Autodesk Inventor part; units mm, degrees
ref_plane "YZ Plane" through (0, 0, 0) normal (1, 0, 0) x (0, 1, 0)
ref_plane "XZ Plane" through (0, 0, 0) normal (0, 1, 0) x (-1, 0, 0)
ref_plane "XY Plane" through (0, 0, 0) normal (0, 0, 1) x (1, 0, 0)
sketch "Sketch1" plane through (0, 0, 0) normal (0, 1, 0) x (-1, 0, 0)
  line L0 (0, 0) -> (325, 0)
  line L1 (325, 0) -> (325, -10)
  line L2 (325, -10) -> (0, -10)
  line L3 (0, -10) -> (0, 0)
  dimension "d0" = 325
  dimension "d1" = 10
extrude "Extrusion1" add sketch "Sketch1" along normal blind 40
sketch "Sketch4" plane through (-325, 0, 0) normal (0, 0, 1) x (1, 0, 0)
  line L0 (325, 0) -> (0, 0)
  line L1 (325, 0) -> (325, 40)
  line L2 (0, 0) -> (325, 0)
  line L3 (325, 0) -> (325, 8)
  line L4 (325, 8) -> (0, 8)
  line L5 (0, 8) -> (0, 0)
  dimension "d34" = 8
extrude "Extrusion3" add sketch "Sketch4" along normal blind 20
sketch "Sketch5" plane through (-325, 40, 0) normal (0, 0, 1) x (1, 0, 0)
  circle A0 centre (320, -25) radius 1.5
  circle A1 centre (320, -15) radius 1.5
  line L0 (325, -32) -> (325, 0)
  line L1 (0, 0) -> (325, 0)
  circle A2 centre (5, -15) radius 1.5
  circle A3 centre (5, -25) radius 1.5
  line L2 (0, -32) -> (0, 0)
  point P0 (325, -40)
  point P1 (325, -27)
  point P2 (0, -27)
  dimension "d39" = 3
  dimension "d40" = 3
  dimension "d41" = 5
  dimension "d42" = 5
  dimension "d43" = 10
  dimension "d44" = 15
  dimension "d45" = 3
  dimension "d46" = 3
  dimension "d47" = 10
  dimension "d48" = 15
  dimension "d49" = 5
  dimension "d50" = 5
extrude "Extrusion4" cut sketch "Sketch5" against normal blind 20
thread "Thread1"
thread "Thread2"
thread "Thread3"
thread "Thread4"
sketch "Sketch8" plane through (0, 0, -10) normal (0, 0, -1) x (-1, 0, 0)
  line L0 (0, 40) -> (325, 40)
  line L1 (12.5, 37) -> (312.5, 37)
  line L2 (312.5, 37) -> (312.5, 0)
  line L3 (312.5, 0) -> (12.5, 0)
  line L4 (12.5, 0) -> (12.5, 37)
  line L5 (0, 0) -> (0, 40)
  line L6 (325, 0) -> (325, 40)
  point P0 (312.5, 18.5)
  dimension "d67" = 300
  dimension "d68" = 37
  dimension "d69" = 12.5
  dimension "d70" = 12.5
  dimension "d71" = 3
extrude "Extrusion5" add sketch "Sketch8" along normal blind 5
sketch "Sketch9" plane through (-325, 40, 0) normal (0, 0, 1) x (1, 0, 0)
  circle A0 centre (57.4993, -19.9899) radius 10
  circle A1 centre (87.4993, -19.9899) radius 10
  circle A2 centre (117.4993, -19.9899) radius 10
  circle A3 centre (147.4993, -19.9899) radius 10
  circle A4 centre (177.4993, -19.9899) radius 10
  circle A5 centre (207.4993, -19.9899) radius 10
  circle A6 centre (237.4993, -19.9899) radius 10
  circle A7 centre (267.4993, -19.9899) radius 10
  line L0 (-0.0007, -39.9899) -> (-0.0007, 0.0101)
  line L1 (324.9993, -39.9899) -> (324.9993, 0.0101)
  line L2 (-0.0007, 0.0101) -> (324.9993, 0.0101)
  point P0 (325, -40)
  dimension "d74" = 20
  dimension "d75" = 20
  dimension "d76" = 20
  dimension "d77" = 20
  dimension "d78" = 20
  dimension "d79" = 20
  dimension "d80" = 20
  dimension "d81" = 20
  dimension "d82" = 30
  dimension "d83" = 30
  dimension "d84" = 30
  dimension "d85" = 30
  dimension "d86" = 30
  dimension "d87" = 30
  dimension "d88" = 30
  dimension "d89" = 57.5
  dimension "d90" = 20
  dimension "d91" = 57.5
extrude "Extrusion6" cut sketch "Sketch9" against normal blind 40
fillet "Fillet2" radius 5 1 edges at (-162.5, 8, 0)
equation "\"d83\" = d82"
equation "\"d84\" = d83"
equation "\"d85\" = d84"
equation "\"d86\" = d85"
equation "\"d87\" = d86"
equation "\"d88\" = d87"
properties part number "chessboard-base-1"
Source: CAD feature listing. Evaluate the final solid. Frame: model axes, mm. A direction names the side the tool comes from. Round coordinates to 2 decimals unless told otherwise and drop trailing zeros. Loops run counter-clockwise (first coordinate to the right, second up) from the corner with the lowest first, then second, coordinate; pieces in that order, holes last. Notation, with made-up numbers: M 74.25,17.5 L 82.25,17.5 A28 cw 82.25,42.5 Z; hole C -30,34 d6. An arc over 180 degrees is marked long. Return JSON: item names as keys, results as strings. Group by question number.
1. Material intervals for line 1 along Y through (x, z) = (-320, -7); line 2 along Z through (x, y) = (-67.5, 10); line 3 along Z through (x, y) = (-294, 13), sorted ascending. Write a range as from..to.
2. Section query A-A on x = -181. Output: boundary loops of the cut face in (y, z).
3. Section query C-C on z = -7. State how many separate pieces and enclosed holes the cut face has, and give its area (3 significant figures).
4. Section query B-B on x = -102. Output: boundary loops of the cut face in (y, z), and give its area (3 significant figures).
5. Mould query, pull axis Y, two halves, no side actions, for faces 3 (the face through (-12.5, 18, -12)), 4 (the face through (-160, 8, 12)), 5 (the face through (-209.67, 10.25, -6.89)). Classes: released by +Y, released by -Y, zero draft, split by the parting line, or undercut.
6. Pin query (flat end, axial travel): pin 1 (2.5 mm diameter, centred on x = -5, y = 25, fed in from +Z); pin 2 (5 mm diameter, centred on x = -214.5, z = 1, fed in from -Y); pin 3 (3.5 mm diameter, centred on x = -320, y = 25, fed in from +Z); pin 4 (10 mm diameter, centred on x = -172, z = 11, fed in from +Y). Return the tip coordinate at first contact, or that it passes through.
7. Reachability of faces 1 (the face through (0, 15, -2)), 2 (the face through (-160, 37, -12)) from +Z, -Z, +X, -X, +Y, -Y: full face, straight path, thin tool, end or side. Return the list, or none.
Checks:
{
 "1": {"line 1": "y = 0..13.5, 16.5..23.5, 26.5..40", "line 2": "z = -15..1", "line 3": "z = -15..0"},
 "2": {"outline": "M 0,-15 L 10.64,-15 L 10.64,0.59 A5 cw 8,5 L 8,20 L 0,20 Z; M 29.38,-15 L 37,-15 L 37,-10 L 40,-10 L 40,0 L 29.38,0 Z"},
 "3": {"separate pieces": "1", "enclosed holes": "12", "area": "10,500 mm²"},
 "4": {"outline": "M 0,-15 L 37,-15 L 37,-10 L 40,-10 L 40,0 L 13,0 A5 cw 8,5 L 8,20 L 0,20 Z", "area": "750 mm²"},
 "5": {"face 3": "zero draft", "face 4": "released by +Y", "face 5": "undercut"},
 "6": {"pin 1": "passes through", "pin 2": "stops at y = 0", "pin 3": "stops at z = 0", "pin 4": "stops at y = 8"},
 "7": {"face 1": "+Z, -Z, +X, +Y, -Y", "face 2": "-Z, +X, -X, +Y"}
}
